Could you check a few things on this model? Use its own coordinates, in mm. A direction names the side the tool comes from. Give positions to 0.01 mm unless a question says otherwise; leave off trailing zeros. Order: outer loops, then holes, each group sorted by start corner. A loop starts at its lowest first (then second) coordinate and runs counter-clockwise, first axis right, second up. Notation, with made-up numbers: M 19.25,-0.5 L 52.25,-0.5 A36 ccw 52.25,38.5 Z; hole C -6,77 d10. An arc over 180 degrees is marked long. Answer in a Markdown table with one row per item. Add a question column.
```python
from build123d import *

# Parameters (mm, degrees)
F1_DEPTH = 9.525
F0_R     = 25.4
F2_DEPTH = 25.4
F0_R_2   = 17.4625
F3_DEPTH = 15.875


with BuildPart() as f1:
    # F0 (on Right) → F1 (new body, symmetric)
    with BuildSketch(Plane.YZ):
        with BuildLine():
            ThreePointArc((-35.9234930565, 42.803092487), (-7.0836883387, 29.4999956791), (4.6830858909, 0))
            ThreePointArc((4.6830858909, 0), (-7.0836883387, -29.4999956791), (-35.9234930565, -42.803092487))
            Line((-35.9234930565, -42.803092487), (144.5501911541, -33.2912941566))
            ThreePointArc((144.5501911541, -33.2912941566), (109.4580858909, 0), (144.5501911541, 33.2912941566))
            Line((144.5501911541, 33.2912941566), (-35.9234930565, 42.803092487))
        make_face()
    extrude(amount=F1_DEPTH, both=True)

    # F0 (on Right) → F2 (join, symmetric)
    with BuildSketch(Plane.YZ):
        with BuildLine():
            ThreePointArc((-35.9234930565, -42.803092487), (-7.0836883387, -29.4999956791), (4.6830858909, 0))
            ThreePointArc((4.6830858909, 0), (-7.0836883387, 29.4999956791), (-35.9234930565, 42.803092487))
            ThreePointArc((-35.9234930565, 42.803092487), (-81.0419141091, 0), (-35.9234930565, -42.803092487))
        make_face()
        with Locations((-38.1794141091, 0)):
            Circle(F0_R, mode=Mode.SUBTRACT)
    extrude(amount=F2_DEPTH, both=True)

    # F0 (on Right) → F3 (join, symmetric)
    with BuildSketch(Plane.YZ):
        with BuildLine():
            ThreePointArc((176.1330858909, 0), (166.981150379, 22.9444410837), (144.5501911541, 33.2912941566))
            ThreePointArc((144.5501911541, 33.2912941566), (109.4580858909, 0), (144.5501911541, -33.2912941566))
            ThreePointArc((144.5501911541, -33.2912941566), (166.981150379, -22.9444410837), (176.1330858909, 0))
        make_face()
        with Locations((142.7955858909, 0)):
            Circle(F0_R_2, mode=Mode.SUBTRACT)
    extrude(amount=F3_DEPTH, both=True)


solid = f1.part
```
1. Thinking about a two-plate mould opening in Y: for faces 1 (the cylindrical face through (-0.222, 150.853, -15.492)), 2 (the flat face through (0.133, 53.05, -38.114)), 3 (the flat face through (-9.525, 53, 1)), 4 (the flat face through (15.875, 157, -14)), which applies, pulls with the +Y half, pulls with the -Y half, needs draft (parallel to the pull), parting line crosses it, or undercut?
2. If I drill on line 1 along Y through (x, z) = (-11.5, -8); line 2 along Y through (x, z) = (-2.5, -14.5); line 3 along Y through (x, z) = (14, 1.5), over which ranges is the centre line in solid material (lowest first)? Write a range as [from, to].
3. Suppose I cut it at A-A on x = 12. List the corners of the cut face in (y, z) for me (1 decimal).
4. For faces 5 (the flat face through (-15.875, 157, -14)), 6 (the cylindrical face through (0.2, 174.6, 10)), 7 (the flat face through (-25.4, -20, -18)), which set-ups out of +Z, -Z, +X, -X, +Y, -Y let a thin tool reach every point of the face, with its end or its side?
5. Will these pins go through, and if not, where does the flat tip stop? P1, Ø5, axis at x = -0.5, z = 14, coming from the -Y side; P2, Ø5, axis at y = 94.5, z = -5.5, coming from the +X side (3 decimals); P3, Ø4, axis at x = -16, z = 6.5, coming from the +Y side.
6. Suppose I cut it at C-C on y = 121.5. List the corners of the cut face in (x, z) for me (3 decimals).
7. Suppose I cut it at D-D on z = 30.5. List the corners of the cut face in (x, y) for me (3 decimals).
8. Suppose I cut it at B-B on z = -8. List the corners of the cut face in (x, y) for me (3 decimals).
Findings below:
| question | item | result |
|---|---|---|
| 1 | face 1 | undercut |
| 1 | face 2 | pulls with the +Y half |
| 1 | face 3 | undercut |
| 1 | face 4 | needs draft |
| 2 | line 1 | [-80.29, -62.29], [-14.07, 3.93], [110.43, 127.27], [158.32, 175.16] |
| 2 | line 2 | [-78.51, -59.03], [-17.32, 133.06], [152.53, 172.81] |
| 2 | line 3 | [-81.02, -63.54], [-12.82, 4.66], [109.49, 125.4], [160.19, 176.1] |
| 3 | outline | C -38.2,0 d85.7; C 142.8,0 d66.7; hole C -38.2,0 d50.8; hole C 142.8,0 d34.9 |
| 4 | face 5 | +Z, -Z, -X, +Y |
| 4 | face 6 | none |
| 4 | face 7 | +Z, -Z, -X, +Y, -Y |
| 5 | P1 | y = -79.47 |
| 5 | P2 | x = 9.525 |
| 5 | P3 | y = 175.83 |
| 6 | outline | M -15.875,-25.649 L -9.525,-25.649 L -9.525,-34.506 L 9.525,-34.506 L 9.525,-25.649 L 15.875,-25.649 L 15.875,25.649 L 9.525,25.649 L 9.525,34.506 L -9.525,34.506 L -9.525,25.649 L -15.875,25.649 Z |
| 7 | outline | M -25.4,-68.295 L 25.4,-68.295 L 25.4,-8.064 L 9.525,-8.064 L 9.525,129.337 L 15.875,129.337 L 15.875,156.254 L -15.875,156.254 L -15.875,129.337 L -9.525,129.337 L -9.525,-8.064 L -25.4,-8.064 Z |
| 8 | outline | M -25.4,-80.289 L 25.4,-80.289 L 25.4,-62.287 L -25.4,-62.287 Z; M -25.4,-14.072 L 25.4,-14.072 L 25.4,3.93 L 9.525,3.93 L 9.525,110.432 L 15.875,110.432 L 15.875,127.273 L -15.875,127.273 L -15.875,110.432 L -9.525,110.432 L -9.525,3.93 L -25.4,3.93 Z; M -15.875,158.318 L 15.875,158.318 L 15.875,175.159 L -15.875,175.159 Z |
